Check sheet for the modelled part. Datum: model origin and axes. Units: mm. Round coordinates to 2 decimals unless told otherwise and drop trailing zeros. Order: outer loops, then holes, each group sorted by start corner. A loop starts at its lowest first (then second) coordinate and runs counter-clockwise, first axis right, second up. Notation, with made-up numbers: (-27.5, 65) -> (-14.5, 65) arc R25 ccw to (-14.5, 92) -> close; hole circle Ø6 at (54.5, 47). An arc over 180 degrees is marked (long way). Answer in a Markdown table with one row per item.
from build123d import *

# Parameters (mm, degrees)
SKETCH004_W     = 166
SKETCH004_H     = 380
PAD002_DEPTH    = 130
SKETCH005_W     = 166
SKETCH005_H     = 380
POCKET002_DEPTH = 120
SKETCH006_W     = 146
SKETCH006_H     = 360
PAD003_DEPTH    = 7.5
SKETCH015_W     = 156
SKETCH015_H     = 370
SKETCH015_W_2   = 146
SKETCH015_H_2   = 360
POCKET008_DEPTH = 2
CHAMFER005_SIZE = 1.5


with BuildPart() as part:
    # Sketch004 → Pad002 (new body)
    with BuildSketch(Plane.XY):
        Rectangle(SKETCH004_W, SKETCH004_H)
    extrude(amount=PAD002_DEPTH)

    # Sketch005 (on Face5 of Pad002) → Pocket002 (cut)
    with BuildSketch(Plane(origin=(0, 0, 0), x_dir=(1, 0, 0), z_dir=(0, 0, -1))):
        Rectangle(SKETCH005_W, SKETCH005_H)
    extrude(amount=-POCKET002_DEPTH, mode=Mode.SUBTRACT)

    # Sketch006 (on Face2 of Pocket002) → Pad003 (join)
    with BuildSketch(Plane(origin=(0, 0, 120), x_dir=(1, 0, 0), z_dir=(0, 0, -1))):
        Rectangle(SKETCH006_W, SKETCH006_H)
    extrude(amount=PAD003_DEPTH)

    # Sketch015 (on Face4 of Pad003) → Pocket008 (cut)
    with BuildSketch(Plane.XY.offset(130)):
        Rectangle(SKETCH015_W, SKETCH015_H)
        Rectangle(SKETCH015_W_2, SKETCH015_H_2, mode=Mode.SUBTRACT)
    extrude(amount=-POCKET008_DEPTH, mode=Mode.SUBTRACT)

    # Chamfer005
    chamfer005_edges = [part.edges().sort_by_distance(p)[0] for p in [
        (83, 0, 120),
        (0, -190, 120),
        (-83, 0, 120),
        (0, 190, 120),
    ]]
    chamfer(chamfer005_edges, length=CHAMFER005_SIZE)


solid = part.part
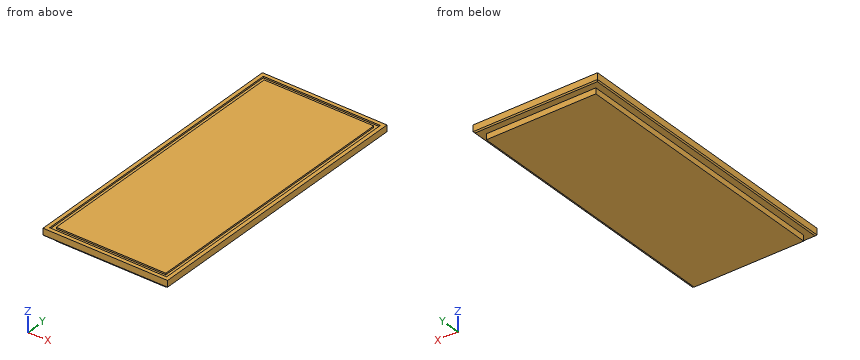
Item 1: Scan lines: line 1 (X direction, y = -58.5, z = 129.25); line 2 (Y direction, x = 4, z = 128.25); line 3 (Y direction, x = -23, z = 115). Record each from-to range of solid material in increasing order. Write a range as [from, to].
Result sheet:
| item | result |
|---|---|
| line 1 | x = [-83, -78], [-73, 73], [78, 83] |
| line 2 | y = [-190, -185], [-180, 180], [185, 190] |
| line 3 | y = [-180, 180] |
Item 2: Cross-section at C-C (z = 116.5). Record the boundary of the cut face in (x, y), and give its area (3 significant figures).
Result sheet:
| item | result |
|---|---|
| outline | (-73, -180) -> (73, -180) -> (73, 180) -> (-73, 180) -> close |
| area | 52,600 mm^2 |
Item 3: Cross-section at B-B (x = -49). Record the boundary of the cut face in (y, z).
Result sheet:
| item | result |
|---|---|
| outline | (-190, 121.5) -> (-188.5, 120) -> (-180, 120) -> (-180, 112.5) -> (180, 112.5) -> (180, 120) -> (188.5, 120) -> (190, 121.5) -> (190, 130) -> (185, 130) -> (185, 128) -> (180, 128) -> (180, 130) -> (-180, 130) -> (-180, 128) -> (-185, 128) -> (-185, 130) -> (-190, 130) -> close |
Item 4: Depth check by flat-ended pin: P1, Ø4, axis at x = 13.5, z = 117.5, coming from the -Y side; P2, Ø4, axis at y = -40.5, z = 116.5, coming from the +X side; P3, Ø6, axis at y = -73.5, z = 115, coming from the -X side; P4, Ø6, axis at x = -2, z = 120.5, coming from the +Y side. Enter the tip coordinate at first touch or a pass-through.
Result sheet:
| item | result |
|---|---|
| P1 | stops at y = -180 |
| P2 | stops at x = 73 |
| P3 | stops at x = -73 |
| P4 | stops at y = 190 |
Item 5: Cross-section at A-A (y = 134). Record the boundary of the cut face in (x, z), and give its area (3 significant figures).
Result sheet:
| item | result |
|---|---|
| outline | (-83, 121.5) -> (-81.5, 120) -> (-73, 120) -> (-73, 112.5) -> (73, 112.5) -> (73, 120) -> (81.5, 120) -> (83, 121.5) -> (83, 130) -> (78, 130) -> (78, 128) -> (73, 128) -> (73, 130) -> (-73, 130) -> (-73, 128) -> (-78, 128) -> (-78, 130) -> (-83, 130) -> close |
| area | 2,730 mm^2 |
